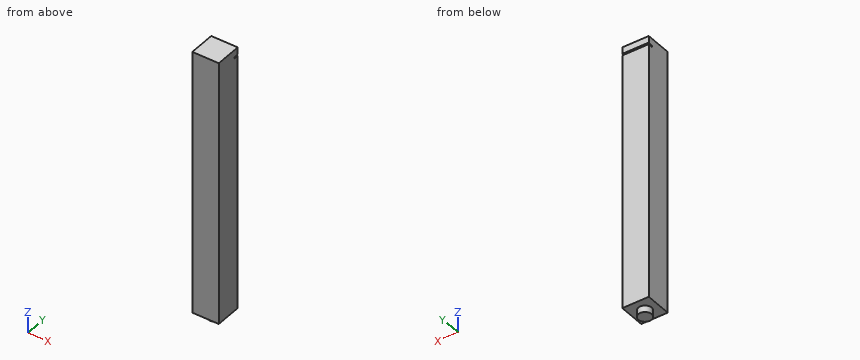
```python
from build123d import *

# Parameters (mm, degrees)
F0_R     = 25.4
F1_DEPTH = 25.4
F2_W     = 101.6
F2_H     = 101.6
F3_DEPTH = 1016
F5_DEPTH = 101.6


with BuildPart() as f1:
    # F0 (on Top) → F1 (new body)
    with BuildSketch(Plane.XY):
        Circle(F0_R)
    extrude(amount=F1_DEPTH)

    # F2 (on face) → F3 (join)
    with BuildSketch(Plane.XY.offset(25.4)):
        Rectangle(F2_W, F2_H)
    extrude(amount=F3_DEPTH)

    # F4 (on face) → F5 (cut)
    with BuildSketch(Plane(origin=(-50.8, 0, 0), x_dir=(0, -1, 0), z_dir=(-1, 0, 0))):
        Polygon((-33.154695, 1013.8156), (-50.8, 1016), (-50.8, 1009.65), (-33.154695, 1007.4656), align=None)
    extrude(amount=-F5_DEPTH, mode=Mode.SUBTRACT)


solid = f1.part
```
Work out the finished part from the listing and answer in its coordinate system (mm). Round coordinates to 2 decimals unless told otherwise and drop trailing zeros. Write each loop counter-clockwise with the first axis right and the second up, starting at its lowest first coordinate (ties: lowest second). Pieces come first, ordered by that corner, then holes. Notation, with made-up numbers: (65.25, 52.25) - (77.25, 52.25) arc R13 ccw to (77.25, 63.25) - close; hole circle Ø3 at (-28, 69). An arc over 180 degrees is marked (long way). Return JSON: item names as keys, results as strings. Group by question number.
Q1. The part is cut by section A-A on x = 39. Write down the section's boundary in (y, z).
Q2. The part is cut by section B-B on x = -16.5. Write down the section's boundary in (y, z), then the cut area to 3 significant figures.
Q3. Find the intervals of material crossed by L1, parallel to Z at x = 38.5, y = 2, in increasing order.
Q4. Each of these flat-tipped pins is pushed along its axis until it touches: pin 1 Ø10 at (x, y) = (-18.5, 12.5) entering from -Z; pin 2 Ø1.9 at (x, z) = (-25.5, 1011.5) entering from +Y; pin 3 Ø1.5 at (x, y) = (-10, -28.5) entering from -Z. Where does it stop, or does it pass through?
Solved:
{
 "1": {"outline": "(-50.8, 25.4) - (50.8, 25.4) - (50.8, 1009.65) - (33.15, 1007.47) - (33.15, 1013.82) - (50.8, 1016) - (50.8, 1041.4) - (-50.8, 1041.4) - close"},
 "2": {"outline": "(-50.8, 25.4) - (-19.31, 25.4) - (-19.31, 0) - (19.31, 0) - (19.31, 25.4) - (50.8, 25.4) - (50.8, 1009.65) - (33.15, 1007.47) - (33.15, 1013.82) - (50.8, 1016) - (50.8, 1041.4) - (-50.8, 1041.4) - close", "area": "104,000 mm²"},
 "3": {"L1": "25.4 to 1041.4"},
 "4": {"pin 1": "z = 0", "pin 2": "y = 33.15", "pin 3": "z = 25.4"}
}
